Could you check a few things on this model? Use its own coordinates, in mm. A direction names the side the tool comes from. Coordinates: 2 decimals unless noted, no trailing zeros. Order: outer loops, then holes, each group sorted by start corner. A loop starts at its lowest first (then second) coordinate and runs counter-clockwise, first axis right, second up. Notation, with made-up numbers: (-38.5, 36.25) - (-29.5, 36.25) arc R17 cw to (-29.5, 40.25) - close; hole circle Ø5 at (80, 54.25). An arc over 180 degrees is marked (long way). One line per item, written item: value.
from build123d import *

# Parameters (mm, degrees)
SKETCH1_R           = 3.175
BOSS_EXTRUDE1_DEPTH = 5
SKETCH2_W           = 110.49
SKETCH2_H           = 15
BOSS_EXTRUDE2_DEPTH = 3.81
SKETCH5_R           = 3.175
BOSS_EXTRUDE3_DEPTH = 5
SKETCH6_W           = 75
SKETCH6_H           = 9.5
CUT_EXTRUDE1_DEPTH  = 6.5
SKETCH7_W           = 12
SKETCH7_H           = 9.5
CUT_EXTRUDE2_DEPTH  = 30.48
BOSS_EXTRUDE4_DEPTH = 19.05
CUT_EXTRUDE3_DEPTH  = 30.48
BOSS_EXTRUDE5_DEPTH = 25.4


with BuildPart() as part:
    # Sketch1 → Boss-Extrude1 (new body)
    with BuildSketch(Plane.XY):
        with BuildLine():
            Line((-47.217391304, 7.923913043), (79.782608696, 7.923913043))
            ThreePointArc((79.782608696, 7.923913043), (95.782608696, -8.076086957), (79.782608696, -24.076086957))
            Line((79.782608696, -24.076086957), (-47.217391304, -24.076086957))
            ThreePointArc((-47.217391304, -24.076086957), (-63.217391304, -8.076086957), (-47.217391304, 7.923913043))
        make_face()
        with Locations((-47.217391304, -8.076086957)):
            Circle(SKETCH1_R, mode=Mode.SUBTRACT)
        with Locations((79.782608696, -8.076086957)):
            Circle(SKETCH1_R, mode=Mode.SUBTRACT)
    extrude(amount=BOSS_EXTRUDE1_DEPTH)

    # Sketch2 → Boss-Extrude2 (add)
    with BuildSketch(Plane.XY.offset(5)):
        with Locations((16.282608696, 0.423913043)):
            Rectangle(SKETCH2_W, SKETCH2_H)
    extrude(amount=BOSS_EXTRUDE2_DEPTH)

    # Sketch5 → Boss-Extrude3 (add)
    with BuildSketch(Plane.XY.offset(8.81)):
        with BuildLine():
            Line((-47.217391304, 7.923913043), (79.782608696, 7.923913043))
            ThreePointArc((79.782608696, 7.923913043), (95.782608696, -8.076086957), (79.782608696, -24.076086957))
            Line((79.782608696, -24.076086957), (-47.217391304, -24.076086957))
            ThreePointArc((-47.217391304, -24.076086957), (-63.217391304, -8.076086957), (-47.217391304, 7.923913043))
        make_face()
        with Locations((-47.217391304, -8.076086957)):
            Circle(SKETCH5_R, mode=Mode.SUBTRACT)
        with Locations((79.782608696, -8.076086957)):
            Circle(SKETCH5_R, mode=Mode.SUBTRACT)
    extrude(amount=BOSS_EXTRUDE3_DEPTH)

    # Sketch6 → Cut-Extrude1 (cut)
    with BuildSketch(Plane(origin=(0, 7.923913043, 0), x_dir=(1, 0, 0), z_dir=(0, 1, 0))):
        with Locations((16.282608696, -6.905)):
            Rectangle(SKETCH6_W, SKETCH6_H)
    extrude(amount=-CUT_EXTRUDE1_DEPTH, mode=Mode.SUBTRACT)

    # Sketch7 → Cut-Extrude2 (cut)
    with BuildSketch(Plane(origin=(0, 1.423913043, 0), x_dir=(1, 0, 0), z_dir=(0, 1, 0))):
        with Locations((-15.217391304, -6.905)):
            Rectangle(SKETCH7_W, SKETCH7_H)
        with Locations((47.782608696, -6.905)):
            Rectangle(SKETCH7_W, SKETCH7_H)
    extrude(amount=-CUT_EXTRUDE2_DEPTH, mode=Mode.SUBTRACT)

    # Sketch10 → Boss-Extrude4 (add)
    with BuildSketch(Plane.XY.offset(13.81)):
        with BuildLine():
            Line((-34.517391304, -20.776086957), (-57.377391304, -20.776086957))
            ThreePointArc((-57.377391304, -20.776086957), (-59.173442529, -20.032138181), (-59.917391304, -18.236086957))
            Line((-59.917391304, -18.236086957), (-59.917391304, 2.083913043))
            ThreePointArc((-59.917391304, 2.083913043), (-59.173442529, 3.879964268), (-57.377391304, 4.623913043))
            Line((-57.377391304, 4.623913043), (-34.517391304, 4.623913043))
            Line((-34.517391304, 4.623913043), (-21.817391304, 4.623913043))
            Line((-21.817391304, 4.623913043), (-21.817391304, -20.776086957))
            Line((-21.817391304, -20.776086957), (-34.517391304, -20.776086957))
        make_face()
    extrude(amount=BOSS_EXTRUDE4_DEPTH)

    # Sketch14 → Cut-Extrude3 (cut)
    with BuildSketch(Plane(origin=(0, 4.623913043, 0), x_dir=(1, 0, 0), z_dir=(0, 1, 0))):
        with BuildLine():
            Line((-59.917391304, -13.81), (-29.183391304, -13.81))
            ThreePointArc((-29.183391304, -13.81), (-29.434604535, -22.554535578), (-35.79555952, -28.560221405))
            Line((-35.79555952, -28.560221405), (-59.917391304, -28.560221405))
            Line((-59.917391304, -28.560221405), (-59.917391304, -13.81))
        make_face()
    extrude(amount=-CUT_EXTRUDE3_DEPTH, mode=Mode.SUBTRACT)

    # Sketch15 → Boss-Extrude5 (add)
    with BuildSketch(Plane.XZ.offset(20.776086957)):
        Polygon((-21.817391304, 13.81), (5.46367495, 13.81), (-21.817391304, 32.86), align=None)
    extrude(amount=-BOSS_EXTRUDE5_DEPTH)


solid = part.part
Item 1: I want a section at A-A on x = 73.5. Please give me the cut outline in (y, z).
Conclusion:
outline: (-24.08, 0) - (7.92, 0) - (7.92, 5) - (-24.08, 5) - close; (-24.08, 8.81) - (7.92, 8.81) - (7.92, 13.81) - (-24.08, 13.81) - close
Item 2: I'm going to push flat-ended pins straight in: pin 1 Ø8.5 at (x, y) = (10, -15.5) entering from +Z; pin 2 Ø8 at (y, z) = (-1.5, 14) entering from -X; pin 3 Ø10 at (y, z) = (-4.5, 27) entering from +X. Where does each tip first touch, or does it pass through?
Conclusion:
pin 1: z = 13.81
pin 2: x = -63.01
pin 3: x = -6.27
Item 3: For faces 1 (the face through (-50.39, -7.94, 2.46)), 2 (the face through (-63.214, -8.428, 2.465)), 3 (the face through (-59.917, -8, 31)), 4 (the face through (63, -7.076, 7)), which set-ups out of +Z, -Z, +X, -X, +Y, -Y let a thin tool reach every point of the face, with its end or its side?
Conclusion:
face 1: -Z
face 2: -Z, -X
face 3: +Z, -X, +Y, -Y
face 4: +X, -X, -Y
Item 4: I want a section at C-C on y = -1.5. Please give me the cut outline in (x, z) (3 decimals).
Conclusion:
outline: (-61.804, 0) - (94.369, 0) - (94.369, 5) - (71.528, 5) - (71.528, 8.81) - (94.369, 8.81) - (94.369, 13.81) - (5.464, 13.81) - (-21.817, 32.86) - (-59.917, 32.86) - (-59.917, 28.56) - (-35.796, 28.56) arc R11.43 cw to (-29.183, 13.81) - (-61.804, 13.81) - (-61.804, 8.81) - (-38.962, 8.81) - (-38.962, 5) - (-61.804, 5) - close; hole (-21.217, 2.155) - (-9.217, 2.155) - (-9.217, 11.655) - (-21.217, 11.655) - close; hole (41.783, 2.155) - (53.783, 2.155) - (53.783, 11.655) - (41.783, 11.655) - close
Item 5: I want a section at D-D on x = -45.5. Please give me the cut outline in (y, z), then the cut area to 3 significant figures.
Conclusion:
outline: (-24.08, 0) - (-10.75, 0) - (-10.75, 5) - (-24.08, 5) - close; (-24.08, 8.81) - (-10.75, 8.81) - (-10.75, 13.81) - (-24.08, 13.81) - close; (-20.78, 28.56) - (4.62, 28.56) - (4.62, 32.86) - (-20.78, 32.86) - close; (-5.41, 0) - (7.92, 0) - (7.92, 5) - (-5.41, 5) - close; (-5.41, 8.81) - (7.92, 8.81) - (7.92, 13.81) - (-5.41, 13.81) - close
area: 376 mm²
Item 6: I want a section at B-B on x = 11. Please give me the cut outline in (y, z) (3 decimals).
Conclusion:
outline: (-24.076, 0) - (7.924, 0) - (7.924, 2.155) - (1.424, 2.155) - (1.424, 11.655) - (7.924, 11.655) - (7.924, 13.81) - (-24.076, 13.81) - (-24.076, 8.81) - (-7.076, 8.81) - (-7.076, 5) - (-24.076, 5) - close
Item 7: If I drill on probe 1 along Z at (x, y) = (-41, -20); probe 2 along X at (y, z) = (-3, 7); probe 3 along Z at (x, y) = (-0.5, 5.5) (3 decimals), over which ranges is the centre line in solid material (lowest first)?
Conclusion:
probe 1: 0 to 5, 8.81 to 13.81, 28.56 to 32.86
probe 2: -38.96 to -21.22, -9.22 to 41.78, 53.78 to 71.53
probe 3: 0 to 2.155, 11.655 to 13.81
Item 8: Thinking about a two-plate mould opening in Z: for faces 5 (the face through (75, -11, 5)), 6 (the face through (7, 3, 2.155)), 7 (the face through (-41, -8, 32.86)), 8 (the face through (-59.154, -20.052, 30.68)), which applies, pulls with the +Z half, pulls with the -Z half, needs draft (parallel to the pull), parting line crosses it, or undercut?
Conclusion:
face 5: undercut
face 6: undercut
face 7: pulls with the +Z half
face 8: needs draft
